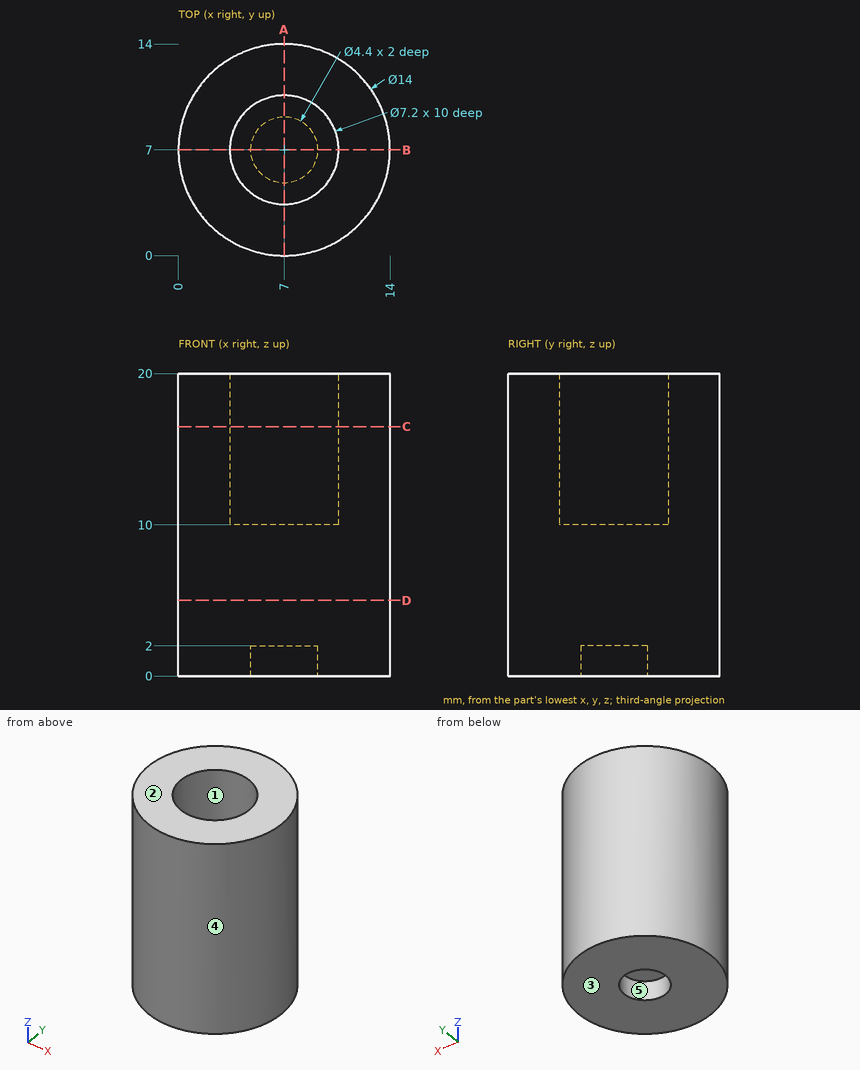
Job drawing, mm, ordinate dimensions from the low corner. One solid piece. A direction names the side the tool comes from. Round coordinates to 2 decimals unless told otherwise and drop trailing zeros. Loops run counter-clockwise (first coordinate to the right, second up) from the corner with the lowest first, then second, coordinate; pieces in that order, holes last. Notation, with made-up numbers: (-12, 15) -> (0, 15) arc R22 ccw to (0, 31) -> close; hole circle Ø11 at (69, -24). An arc over 180 degrees is marked (long way). Use CSV: the item, a comma, the result in double quotes. Start each with the question number.
Q1. Which spindle directions (+Z, -Z, +X, -X, +Y, -Y) get a long thin tool onto all of the face, cutting with end or side? Do the marked faces 1 and 2. Say none if no direction does.
Q2. Mould opens along X. For the marked faces 3, 4 and 5 say: +X half, -X half, draft (parallel to the pull), parting line (faces both ways), or undercut.
Q3. Flat gauge pins, fed straight in: pin 1 Ø5.5 at (x, y) = (7, 7) entering from +Z; pin 2 Ø1 at (y, z) = (8.5, 4.5) entering from -X; pin 3 Ø6 at (x, z) = (3, 4.5) entering from +Y. Where does each tip first touch, or does it go through?
Q4. Saw through at C-C on z = 16.5. Give the cut face in (x, y).
Q5. Saw through at D-D on z = 5. Give the cut face in (x, y).
Q6. Saw through at A-A on x = 7. Give the cut face in (y, z).
Q7. Drill centre lines: L1, parallel to Y at x = 7, z = 1.5; L2, parallel to Z at x = 5, y = 7.5; L3, parallel to X at y = 1, z = 15.75. Where is each one in solid material? Low to high.
Solutions:
1,face 1,"+Z"
1,face 2,"+Z, +X, -X, +Y, -Y"
2,face 3,"draft"
2,face 4,"parting line"
2,face 5,"undercut"
3,pin 1,"stops at z = 10"
3,pin 2,"stops at x = 0.07"
3,pin 3,"stops at y = 13.93"
4,outline,"circle Ø14 at (7, 7); hole circle Ø7.2 at (7, 7)"
5,outline,"circle Ø14 at (7, 7)"
6,outline,"(0, 0) -> (4.8, 0) -> (4.8, 2) -> (9.2, 2) -> (9.2, 0) -> (14, 0) -> (14, 20) -> (10.6, 20) -> (10.6, 10) -> (3.4, 10) -> (3.4, 20) -> (0, 20) -> close"
7,L1,"y = 0 to 4.8, 9.2 to 14"
7,L2,"z = 2 to 10"
7,L3,"x = 3.39 to 10.61"
